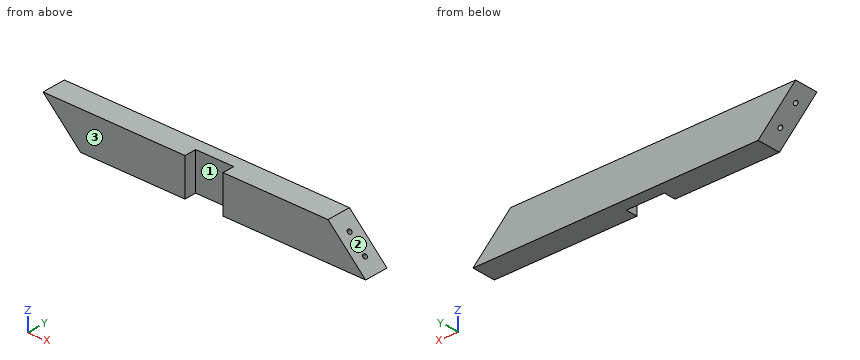
from build123d import *

# Parameters (mm, degrees)
F0_W     = 44
F0_H     = 69
F1_DEPTH = 593
F2_SIZE  = 68.99999
F4_D     = 8
F4_DEPTH = 20
F4_TIP   = 2.4034424761
F5_SIZE  = 68.99999
F7_D     = 8
F7_DEPTH = 20
F7_TIP   = 2.4034424761
F8_W     = 70
F8_H     = 69
F9_DEPTH = 22


# Not quite as in the source:
# - a fillet or chamfer is up to 0.001 mm smaller than in the source, because OpenCascade refuses the exact size


with BuildPart() as f1:
    # F0 (on Right) → F1 (new body)
    with BuildSketch(Plane.YZ):
        with Locations((2.3388881236, 4.4023249735)):
            Rectangle(F0_W, F0_H)
    extrude(amount=F1_DEPTH)

    # F2 (size 69 in the source; OpenCascade refuses exactly that, so slightly less here)
    f2_edges = [f1.edges().sort_by_distance(p)[0] for p in [
        (0, 2.338888, -30.097675),
    ]]
    chamfer(f2_edges, length=F2_SIZE)

    # F4
    with Locations(Plane(origin=(19.4511624867, 0, 19.4511624867), x_dir=(0, -1, 0), z_dir=(-0.7071067812, 0, -0.7071067812))):
        with Locations((-2.3388881236, 0), (-2.3388881236, -40)):
            Hole(F4_D / 2, depth=F4_DEPTH)
            with Locations((0, 0, -(F4_DEPTH + F4_TIP / 2))):  # 118° drill point
                Cone(0, F4_D / 2, F4_TIP, mode=Mode.SUBTRACT)

    # F5 (size 69 in the source; OpenCascade refuses exactly that, so slightly less here)
    f5_edges = [f1.edges().sort_by_distance(p)[0] for p in [
        (593, 2.338888, 38.902325),
    ]]
    chamfer(f5_edges, length=F5_SIZE)

    # F7
    with Locations(Plane(origin=(281.4511624867, 0, 281.4511624867), x_dir=(0, 1, 0), z_dir=(0.7071067812, 0, 0.7071067812))):
        with Locations((1.8450106473, -371.8575412992), (1.8450106473, -411.8575412992)):
            Hole(F7_D / 2, depth=F7_DEPTH)
            with Locations((0, 0, -(F7_DEPTH + F7_TIP / 2))):  # 118° drill point
                Cone(0, F7_D / 2, F7_TIP, mode=Mode.SUBTRACT)

    # F8 (on face) → F9 (cut)
    with BuildSketch(Plane.XZ.offset(19.6611118764)):
        with Locations((296, 4.4023249735)):
            Rectangle(F8_W, F8_H)
    extrude(amount=-F9_DEPTH, mode=Mode.SUBTRACT)


solid = f1.part
Check sheet for the modelled part. Datum: model origin and axes. Units: mm. Face numbers are marked on the shaded views. Round coordinates to 2 decimals unless told otherwise and drop trailing zeros. Loops run counter-clockwise (first coordinate to the right, second up) from the corner with the lowest first, then second, coordinate; pieces in that order, holes last. Notation, with made-up numbers: (67, -13.75) - (88, -13.75) arc R22 ccw to (88, 2.25) - close; hole circle Ø1 at (-40, -12). An arc over 180 degrees is marked (long way). Answer as CSV lines item,"result". Start each with the question number.
Item 1: Section check B-B (x = 267). Record the boundary of the cut face in (y, z).
Item 2: Scan lines: line 1 (X direction, y = 1.5, z = 29.5); line 2 (X direction, y = -16.5, z = 2.5); line 3 (X direction, y = -16, z = -13.5). Record each from-to range of solid material in increasing order. Write a range as [from, to].
Item 3: Depth check by flat-ended pin: P1, Ø1.5, axis at y = 8.5, z = 20, coming from the -X side; P2, Ø2, axis at y = 8, z = 1.5, coming from the -X side; P3, Ø6.5, axis at y = -3.5, z = 2, coming from the +X side. Enter the tip coordinate at first touch or a pass-through.
Item 4: Release check for a two-part mould opening along X. For the marked faces 1, 2 and 3 record: +X half, -X half, draft (parallel to the pull), parting line (faces both ways), or undercut.
Report:
1,outline,"(2.34, -30.1) - (24.34, -30.1) - (24.34, 38.9) - (2.34, 38.9) - close"
2,line 1,"x = [9.4, 23.97], [35.03, 261], [331, 533.4]"
2,line 2,"x = [36.4, 261], [331, 560.4]"
2,line 3,"x = [52.4, 261], [331, 576.4]"
3,P1,"stops at x = 18.15"
3,P2,"stops at x = 36.4"
3,P3,"stops at x = 564.15"
4,face 1,"undercut"
4,face 2,"+X half"
4,face 3,"draft"
